Work out the finished part from the listing and answer in its coordinate system (mm). A direction names the side the tool comes from. Round coordinates to 2 decimals unless told otherwise and drop trailing zeros. Order: outer loops, then holes, each group sorted by start corner. A loop starts at its lowest first (then second) coordinate and runs counter-clockwise, first axis right, second up. Notation, with made-up numbers: (-18.5, -17.5) -> (34.5, -17.5) arc R5 ccw to (34.5, -13.5) -> close; hole circle Ø9 at (75.5, 75.5). An arc over 180 degrees is marked (long way). Use a Markdown table: item, result. Add a question column.
Item 1: A cutting plane is placed at A-A, the plane z = -2.5. Determine the outline of the cut face in (x, y).
Item 2: A cutting plane is placed at D-D, the plane y = 11. Determine the outline of the cut face in (x, z), plus the area to 3 significant figures.
Item 3: Find the intervals of material crossed by L1, parallel to Z at x = -4.5, y = 4.5; L2, parallel to X at y = 2.25, z = -0.75; L3, parallel to X at y = 6, z = -4, in increasing order. Write a range as [from, to].
Item 4: For a pull along X with two mould halves and no side action, classify faces 6 (the flat face through (-4.5, 4.8, 0)), 7 (the flat face through (-5.4, 0, 0.1)), 8 (the cylindrical face through (6, 6, 1)), 9 (the flat face through (-9, 6, -1)) as +X half, -X half, draft (parallel to the pull), parting line (faces both ways), or undercut.
Item 5: A cutting plane is placed at C-C, the plane x = 4.25. Determine the outline of the cut face in (y, z).
Item 6: A cutting plane is placed at B-B, the plane y = 4.75. Determine the outline of the cut face in (x, z).
Item 7: A tool of negligible diameter and unlimited length cuts with its end or side. For faces 1 (the flat face through (-5, 6, -1)), 2 (the flat face through (-7, 6, -3)), 3 (the flat face through (-1, 6, 2)), 4 (the flat face through (-8.5, 6.1, 0)), 5 (the flat face through (-6, 12, 0)), from which of +Z, -Z, +X, -X, +Y, -Y can it reach the whole face along a straight path? Write none if from no direction.
Item 8: A flat-ended cylindrical pin translates along its axis: P1, Ø1.2, axis at x = -6.5, y = 8, coming from the -Z side. Find the tip coordinate at first contact, or state that the pin passes through.
from build123d import *

# Parameters (mm, degrees)
SKETCH1_R           = 4.5
SKETCH1_W           = 8
SKETCH1_H           = 12
BOSS_EXTRUDE1_DEPTH = 2
BOSS_EXTRUDE2_DEPTH = 4.5
BOSS_EXTRUDE3_DEPTH = 5
SKETCH3_W           = 1
SKETCH3_H           = 12
SKETCH3_W_2         = 3
BOSS_EXTRUDE4_DEPTH = 3


with BuildPart() as part:
    # Sketch1 → Boss-Extrude1 (new body)
    with BuildSketch(Plane.XY):
        with Locations((0, 6)):
            Circle(SKETCH1_R)
        with Locations((-4, 6)):
            Rectangle(SKETCH1_W, SKETCH1_H)
        with BuildLine():
            ThreePointArc((0, 10.5), (-4.5, 6), (0, 1.5))
            Line((0, 1.5), (0, 5.5))
            ThreePointArc((0, 5.5), (-0.5, 6), (0, 6.5))
            Line((0, 6.5), (0, 10.5))
        make_face()
        with BuildLine():
            Line((0, 5.5), (0, 1.5))
            ThreePointArc((0, 1.5), (3.181980515, 2.818019485), (4.5, 6))
            ThreePointArc((4.5, 6), (3.181980515, 9.181980515), (0, 10.5))
            Line((0, 10.5), (0, 6.5))
            ThreePointArc((0, 6.5), (0.353553391, 6.353553391), (0.5, 6))
            ThreePointArc((0.5, 6), (0.353553391, 5.646446609), (0, 5.5))
        make_face()
        with BuildLine():
            Line((0, 0), (0, 12))
            ThreePointArc((0, 12), (6, 6), (0, 0))
        make_face()
    extrude(amount=BOSS_EXTRUDE1_DEPTH)



with BuildPart() as body_2:
    # Sketch1_3 → Boss-Extrude2 (new body)
    with BuildSketch(Plane.XY):
        with BuildLine():
            ThreePointArc((0, 6.5), (-0.5, 6), (0, 5.5))
            Line((0, 5.5), (0, 6.5))
        make_face()
        with BuildLine():
            Line((0, 6.5), (0, 5.5))
            ThreePointArc((0, 5.5), (0.353553391, 5.646446609), (0.5, 6))
            ThreePointArc((0.5, 6), (0.353553391, 6.353553391), (0, 6.5))
        make_face()
        with BuildLine():
            ThreePointArc((0, 10.5), (-4.5, 6), (0, 1.5))
            Line((0, 1.5), (0, 5.5))
            ThreePointArc((0, 5.5), (-0.5, 6), (0, 6.5))
            Line((0, 6.5), (0, 10.5))
        make_face()
        with BuildLine():
            Line((0, 5.5), (0, 1.5))
            ThreePointArc((0, 1.5), (3.181980515, 2.818019485), (4.5, 6))
            ThreePointArc((4.5, 6), (3.181980515, 9.181980515), (0, 10.5))
            Line((0, 10.5), (0, 6.5))
            ThreePointArc((0, 6.5), (0.353553391, 6.353553391), (0.5, 6))
            ThreePointArc((0.5, 6), (0.353553391, 5.646446609), (0, 5.5))
        make_face()
    extrude(amount=-BOSS_EXTRUDE2_DEPTH)


with BuildPart() as part_1:
    add(part.part)

    add(body_2.part)  # Boss-Extrude3 merges body 2
    # Sketch1_4 → Boss-Extrude3 (add)
    with BuildSketch(Plane.XY):
        with BuildLine():
            ThreePointArc((0, 6.5), (-0.5, 6), (0, 5.5))
            Line((0, 5.5), (0, 6.5))
        make_face()
        with BuildLine():
            Line((0, 6.5), (0, 5.5))
            ThreePointArc((0, 5.5), (0.353553391, 5.646446609), (0.5, 6))
            ThreePointArc((0.5, 6), (0.353553391, 6.353553391), (0, 6.5))
        make_face()
    extrude(amount=-BOSS_EXTRUDE3_DEPTH)

    # Sketch3 → Boss-Extrude4 (add)
    with BuildSketch(Plane(origin=(0, 0, 0), x_dir=(-1, 0, 0), z_dir=(0, 0, -1))):
        with Locations((8.5, 6)):
            Rectangle(SKETCH3_W, SKETCH3_H)
        with Locations((6.5, 6)):
            Rectangle(SKETCH3_W_2, SKETCH3_H)
    extrude(amount=BOSS_EXTRUDE4_DEPTH)


solid = part_1.part
Reported:
| question | item | result |
|---|---|---|
| 1 | outline | (-9, 0) -> (-5, 0) -> (-5, 12) -> (-9, 12) -> close; circle Ø9 at (0, 6) |
| 2 | outline | (-9, -3) -> (-5, -3) -> (-5, 0) -> (3.32, 0) -> (3.32, 2) -> (-8, 2) -> (-8, 0) -> (-9, 0) -> close |
| 2 | area | 34.6 mm² |
| 3 | L1 | [0, 2] |
| 3 | L2 | [-9, -5], [-2.49, 2.49] |
| 3 | L3 | [-4.5, 4.5] |
| 4 | face 6 | undercut |
| 4 | face 7 | draft |
| 4 | face 8 | +X half |
| 4 | face 9 | -X half |
| 5 | outline | (1.76, 0) -> (4.52, 0) -> (4.52, -4.5) -> (7.48, -4.5) -> (7.48, 0) -> (10.24, 0) -> (10.24, 2) -> (1.76, 2) -> close |
| 6 | outline | (-9, -3) -> (-5, -3) -> (-5, 0) -> (-4.32, 0) -> (-4.32, -4.5) -> (4.32, -4.5) -> (4.32, 0) -> (5.87, 0) -> (5.87, 2) -> (-8, 2) -> (-8, 0) -> (-9, 0) -> close |
| 7 | face 1 | -Z, +Y, -Y |
| 7 | face 2 | -Z, -X, +Y, -Y |
| 7 | face 3 | +Z, +X, -X, +Y, -Y |
| 7 | face 4 | +Z, -X, +Y, -Y |
| 7 | face 5 | +Z, -Z, +X, -X, +Y |
| 8 | P1 | z = -3 |
